```python
from build123d import *

# Parameters (mm, degrees)
F0_W     = 101.6
F0_H     = 76.2
F1_DEPTH = 25.4
F2_R     = 38.09999
F3_R     = 19.05
F4_DEPTH = 25.401
F5_W     = 25.4
F5_H     = 76.2
F6_DEPTH = 76.2
F7_W     = 25.4
F7_H     = 25.4
F8_DEPTH = 25.4


# Not quite as in the source:
# - a fillet or chamfer is up to 0.001 mm smaller than in the source, because OpenCascade refuses the exact size


with BuildPart() as f1:
    # F0 (on Top) → F1 (new body)
    with BuildSketch(Plane.XY):
        Rectangle(F0_W, F0_H)
    extrude(amount=F1_DEPTH)

    # F2 (radius 38.1 in the source; OpenCascade refuses exactly that, so slightly less here)
    f2_edges = [f1.edges().sort_by_distance(p)[0] for p in [
        (50.8, -38.1, 12.7),
        (50.8, 38.1, 12.7),
    ]]
    fillet(f2_edges, radius=F2_R)

    # F3 (on Top) → F4 (cut, through all)
    with BuildSketch(Plane.XY):
        Circle(F3_R)
    extrude(amount=F4_DEPTH, mode=Mode.SUBTRACT)

    # F5 (on face) → F6 (join)
    with BuildSketch(Plane.XY.offset(25.4)):
        with Locations((-63.5, 0)):
            Rectangle(F5_W, F5_H)
    extrude(amount=-F6_DEPTH)

    # F7 (on face) → F8 (cut)
    with BuildSketch(Plane.YZ.offset(-50.8)):
        with Locations((25.4, -38.1)):
            Rectangle(F7_W, F7_H)
    extrude(amount=-F8_DEPTH, mode=Mode.SUBTRACT)


solid = f1.part
```
Source: CAD feature listing. Evaluate the final solid. Frame: model axes, mm. A direction names the side the tool comes from. Coordinates: 2 decimals unless noted, no trailing zeros. Loops run counter-clockwise (first coordinate to the right, second up) from the corner with the lowest first, then second, coordinate; pieces in that order, holes last. Notation, with made-up numbers: (-21.5, -15.75) -> (-17.5, -15.75) arc R11 ccw to (-17.5, -7.75) -> close; hole circle Ø10 at (42.25, -37.75). An arc over 180 degrees is marked (long way). One line per item, written item: value. Start each with the question number.
Q1. Section query A-A, the plane x = 0. Return the cut outline in (y, z), and give its area (3 significant figures).
Q2. Set-up query: faces 5 (the face through (-50.8, -9, -25)), 6 (the face through (-63, 25, -25.4)), 7 (the face through (-76.2, -1, -12)). Return all of +Z, -Z, +X, -X, +Y, -Y with unobstructed straight access to the full face (end or side cutting, diameter ignored); none if empty.
Q3. Contact query for flat-ended pins moving along their axis: P1, Ø4, axis at x = 36, z = 5.5, coming from the +Y side; P2, Ø4, axis at y = 8, z = -42, coming from the +X side; P3, Ø12.5, axis at x = -65.5, z = -41.5, coming from the +Y side; P4, Ø12, axis at x = 28, z = -7, coming from the -Y side. Output: stop coordinate, or through.
Q4. Mould query, pull axis Y, two halves, no side actions, for faces 1 (the face through (-12, 17, 0)), 2 (the face through (-63, 12.7, -38)), 3 (the face through (39.34, -27.24, 12.88)), 4 (the face through (-15.12, -11.59, 12.52)). Classes: pulls with the +Y half, pulls with the -Y half, needs draft (parallel to the pull), parting line crosses it, or undercut.
Q5. Line query: line 1 along Y through (x, z) = (0, 5.75); line 2 along X through (y, z) = (-1.5, -4.5); line 3 along Y through (x, z) = (2, 9.5). Output: solid intervals per line, ascending.
Q6. Section query D-D, the plane z = -21. Return the cut outline in (x, y), and give its area (3 significant figures).
Q7. Section query B-B, the plane y = 16. Return the cut outline in (x, z), and give its area (3 significant figures).
Results:
1. outline: (-38.1, 0) -> (-19.05, 0) -> (-19.05, 25.4) -> (-38.1, 25.4) -> close; (19.05, 0) -> (38.1, 0) -> (38.1, 25.4) -> (19.05, 25.4) -> close
1. area: 968 mm^2
2. face 5: -Z, +X, +Y, -Y
2. face 6: -Z, +X, -X, +Y
2. face 7: +Z, -Z, -X, +Y, -Y
3. P1: y = 31.59
3. P2: x = -50.8
3. P3: y = 12.7
3. P4: through
4. face 1: needs draft
4. face 2: pulls with the +Y half
4. face 3: pulls with the -Y half
4. face 4: undercut
5. line 1: -38.1 to -19.05, 19.05 to 38.1
5. line 2: -76.2 to -50.8
5. line 3: -38.1 to -18.94, 18.94 to 38.1
6. outline: (-76.2, -38.1) -> (-50.8, -38.1) -> (-50.8, 38.1) -> (-76.2, 38.1) -> close
6. area: 1,940 mm^2
7. outline: (-76.2, -25.4) -> (-50.8, -25.4) -> (-50.8, 0) -> (-10.34, 0) -> (-10.34, 25.4) -> (-76.2, 25.4) -> close; (10.34, 0) -> (47.28, 0) -> (47.28, 25.4) -> (10.34, 25.4) -> close
7. area: 3,260 mm^2
